The listing builds one solid part. Answer for the finished solid, in the listing's coordinates (mm). Give positions to 0.01 mm unless a question says otherwise; leave off trailing zeros. Write each loop counter-clockwise with the first axis right and the second up, starting at its lowest first coordinate (ties: lowest second). Pieces come first, ordered by that corner, then holes. Notation, with made-up numbers: M 50,47 L 58,47 A15 cw 58,75 Z; hole C 4.5,66 d8. An arc over 180 degrees is marked long. Answer as a JSON object with one key per item and string values.
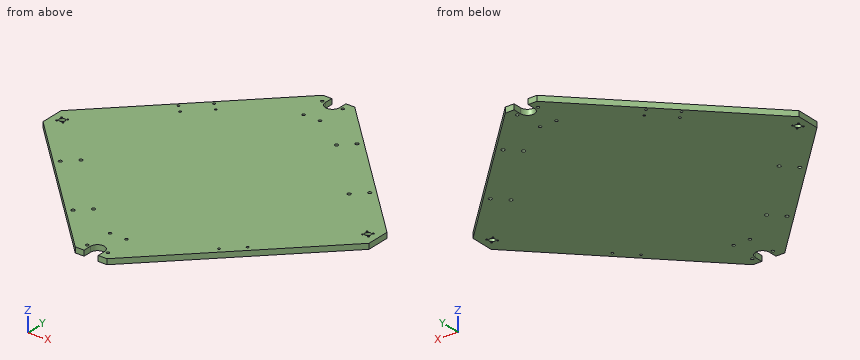
Autodesk Inventor part; units mm, degrees
ref_plane "Work Plane1" through (0, 0, 0) normal (0, 0, 1) x (1, 0, 0)
ref_plane "YZ Plane" through (0, 0, 0) normal (1, 0, 0) x (0, 1, 0)
ref_plane "XZ Plane" through (0, 0, 0) normal (0, 1, 0) x (-1, 0, 0)
sketch "Sketch2" plane through (0, 0, 0) normal (0, 0, 1) x (1, 0, 0)
  circle A0 centre (0, 277.5) radius 8 construction
  circle A1 centre (0, 277.5) radius 13
  circle A2 centre (0, 277.5) radius 10.5 construction
  line L0 (25, 287.5) -> (-25, 287.5) construction
  line L1 (-25, 287.5) -> (-25, 222.5) construction
  line L2 (-25, 222.5) -> (25, 222.5) construction
  line L3 (25, 222.5) -> (25, 287.5) construction
  circle A3 centre (15, 228.5) radius 2.7
  circle A4 centre (-15, 228.5) radius 2.7
  circle A5 centre (-19, 277.5) radius 2.7
  circle A6 centre (19, 277.5) radius 2.7
  circle A7 centre (0, -277.5) radius 8 construction
  circle A8 centre (0, -277.5) radius 13
  circle A9 centre (0, -277.5) radius 10.5 construction
  line L4 (25, -287.5) -> (-25, -287.5) construction
  line L5 (-25, -287.5) -> (-25, -222.5) construction
  line L6 (-25, -222.5) -> (25, -222.5) construction
  line L7 (25, -222.5) -> (25, -287.5) construction
  circle A10 centre (-15, -228.5) radius 2.7
  circle A11 centre (15, -228.5) radius 2.7
  circle A12 centre (-19, -277.5) radius 2.7
  circle A13 centre (19, -277.5) radius 2.7
  line L8 (10.5, -277.5) -> (10.5, -287.5) construction
  line L9 (-10.5, -277.5) -> (-10.5, -287.5) construction
  line L10 (10.5, 277.5) -> (10.5, 287.5) construction
  line L11 (-10.5, 277.5) -> (-10.5, 287.5) construction
  circle A14 centre (281.7, 0) radius 5.25
  circle A15 centre (-281.7, 0) radius 5.25
  line L12 (0, -321.7336) -> (321.7336, 0)
  line L13 (321.7336, 0) -> (0, 321.7336)
  line L14 (0, 321.7336) -> (-321.7336, 0)
  line L15 (-321.7336, 0) -> (0, -321.7336)
  line L16 (0, -321.7336) -> (0, 321.7336) construction
  line L17 (321.7336, 0) -> (-321.7336, 0) construction
  line L18 (0, -321.7336) -> (455, -321.7336) construction
  line L19 (300.5, 21.2336) -> (300.5, -21.2336)
  line L20 (-300.5, 21.2336) -> (-300.5, -21.2336)
  line L21 (-24.2336, 297.5) -> (24.2336, 297.5) construction
  line L22 (-29.2336, 292.5) -> (29.2336, 292.5)
  line L23 (-24.2336, -297.5) -> (24.2336, -297.5) construction
  line L24 (-29.2336, -292.5) -> (29.2336, -292.5)
  line L25 (-9.5, 297.5) -> (-3.976, 284.442) construction
  line L26 (9.5, 297.5) -> (3.976, 284.442) construction
  line L27 (-14.929, 297.5) -> (-9.9883, 285.8207)
  line L28 (14.929, 297.5) -> (9.9883, 285.8207)
  line L29 (-9.5, -297.5) -> (-3.976, -284.442) construction
  line L30 (9.5, -297.5) -> (3.976, -284.442) construction
  line L31 (14.929, -297.5) -> (9.9883, -285.8207)
  line L32 (-14.929, -297.5) -> (-9.9883, -285.8207)
  line L33 (13, 277.5) -> (13, 292.5)
  line L34 (-13, 277.5) -> (-13, 292.5)
  line L35 (-13, -277.5) -> (-13, -292.5)
  line L36 (13, -277.5) -> (13, -292.5)
  line L37 (281.7, 0) -> (287.3569, 5.6569) construction
  line L38 (281.7, 0) -> (289.7, 0) construction
  circle A16 centre (287.3569, 5.6569) radius 1.6
  circle A17 centre (276.0431, 5.6569) radius 1.6
  circle A18 centre (276.0431, -5.6569) radius 1.6
  circle A19 centre (287.3569, -5.6569) radius 1.6
  line L39 (-281.7, 0) -> (-287.3569, 5.6569) construction
  circle A20 centre (-287.3569, 5.6569) radius 1.6
  circle A21 centre (-287.3569, -5.6569) radius 1.6
  circle A22 centre (-276.0431, -5.6569) radius 1.6
  circle A23 centre (-276.0431, 5.6569) radius 1.6
  point P0 (0, 0)
  point P1 (-12.8138, -292.5)
  point P2 (12.8138, -292.5)
  point P3 (12.8138, 292.5)
  point P4 (-12.8138, 292.5)
  point P5 (300.5, 292.5)
  point P6 (300.5, -292.5)
  point P7 (-300.5, -292.5)
  point P8 (-300.5, 292.5)
  dimension "d349" = 450
  dimension "d350" = 45
  dimension "d353" = 40
  dimension "d354" = 10
  dimension "d355" = 10
  dimension "d358" = 40
  dimension "d359" = 10
  dimension "d360" = 10
  dimension "d361" = 6.2
  dimension "d362" = 75
  dimension "d363" = 5
  dimension "d364" = 6.2
  dimension "d365" = 5
  dimension "d366" = 75
  dimension "d367" = 450
  dimension "d368" = 45
  dimension "d369" = 6.2
  dimension "d370" = 5
  dimension "d371" = 75
  dimension "d372" = 6.2
  dimension "d373" = 5
  dimension "d374" = 75
  dimension "d256" = 16
  dimension "d257" = 0
  dimension "d258" = 277.5
  dimension "d259" = 26
  dimension "d260" = 21
  dimension "d261" = 50
  dimension "d262" = 10
  dimension "d263" = 65
  dimension "d265" = 50
  dimension "d266" = 25
  dimension "d267" = 5.4
  dimension "d268" = 5.4
  dimension "d269" = 5.4
  dimension "d270" = 5.4
  dimension "d271" = 6
  dimension "d272" = 10
  dimension "d273" = 6
  dimension "d274" = 10
  dimension "d275" = 6
  dimension "d276" = 10
  dimension "d277" = 6
  dimension "d278" = 10
  dimension "d279" = 0
  dimension "d280" = 277.5
  dimension "d281" = 26
  dimension "d282" = 16
  dimension "d283" = 21
  dimension "d284" = 50
  dimension "d285" = 10
  dimension "d286" = 65
  dimension "d287" = 25
  dimension "d288" = 5.4
  dimension "d289" = 5.4
  dimension "d290" = 5.4
  dimension "d291" = 5.4
  dimension "d292" = 6
  dimension "d293" = 10
  dimension "d294" = 6
  dimension "d295" = 10
  dimension "d296" = 10
  dimension "d297" = 6
  dimension "d298" = 10
  dimension "d299" = 6
  dimension "d300" = 10.5
  dimension "d301" = 0
  dimension "d302" = 281.7
  dimension "d310" = 10.5
  dimension "d311" = 0
  dimension "d312" = 281.7
  dimension "d320" = 455
  dimension "d321" = 45
  dimension "d322" = 455
  dimension "d323" = 18.8
  dimension "d324" = 18.8
  dimension "d325" = 20
  dimension "d326" = 15
  dimension "d327" = 20
  dimension "d328" = 15
  dimension "d329" = 67.07
  dimension "d330" = 67.07
  dimension "d331" = 9.5
  dimension "d332" = 9.5
  dimension "d333" = 67.07
  dimension "d334" = 67.07
ref_plane "Work Plane1" through (0, 0, 0) normal (0, 0, 1) x (1, 0, 0)
sketch "Sketch3" plane through (0, 0, 0) normal (0, 0, 1) x (1, 0, 0)
  line L0 (-159.099, -159.099) -> (159.099, 159.099)
  line L1 (-159.099, -159.099) -> (290.901, -159.099) construction
  line L2 (279.2843, 34.9264) -> (34.9264, 279.2843)
  line L3 (34.9264, 279.2843) -> (6.6421, 251)
  line L4 (6.6421, 251) -> (251, 6.6421)
  line L5 (251, 6.6421) -> (279.2843, 34.9264)
  line L6 (279.2843, 34.9264) -> (6.6421, 251) construction
  line L7 (34.9264, 279.2843) -> (251, 6.6421) construction
  circle A0 centre (19, 277.5) radius 2.7
  circle A1 centre (15, 228.5) radius 2.7
  line L8 (-34.9264, -279.2843) -> (-279.2843, -34.9264)
  line L9 (-279.2843, -34.9264) -> (-251, -6.6421)
  line L10 (-251, -6.6421) -> (-6.6421, -251)
  line L11 (-6.6421, -251) -> (-34.9264, -279.2843)
  line L12 (-34.9264, -279.2843) -> (-251, -6.6421) construction
  line L13 (-279.2843, -34.9264) -> (-6.6421, -251) construction
  circle A2 centre (-15, -228.5) radius 2.7
  circle A3 centre (-19, -277.5) radius 2.7
  circle A4 centre (-79.3236, -185.3896) radius 3.1
  circle A5 centre (-100.5368, -206.6028) radius 3.1
  circle A6 centre (-185.3896, -79.3236) radius 3.1
  circle A7 centre (-206.6028, -100.5368) radius 3.1
  line L14 (-159.099, 159.099) -> (159.099, -159.099)
  line L15 (300.5, -21.2336) -> (29.2336, -292.5)
  line L16 (-159.099, 159.099) -> (290.901, 159.099) construction
  circle A8 centre (206.6028, 100.5368) radius 3.1
  circle A9 centre (185.3896, 79.3236) radius 3.1
  circle A10 centre (100.5368, 206.6028) radius 3.1
  circle A11 centre (79.3236, 185.3896) radius 3.1
  point P0 (0, 0)
  point P1 (142.9632, 142.9632)
  point P2 (-142.9632, -142.9632)
  point P3 (29.2336, -292.5)
  dimension "d349" = 450
  dimension "d350" = 45
  dimension "d353" = 40
  dimension "d354" = 10
  dimension "d355" = 10
  dimension "d358" = 40
  dimension "d359" = 10
  dimension "d360" = 10
  dimension "d361" = 6.2
  dimension "d362" = 75
  dimension "d363" = 5
  dimension "d364" = 6.2
  dimension "d365" = 5
  dimension "d366" = 75
  dimension "d367" = 450
  dimension "d368" = 45
  dimension "d369" = 6.2
  dimension "d370" = 5
  dimension "d371" = 75
  dimension "d372" = 6.2
  dimension "d373" = 5
  dimension "d374" = 75
extrude "Extrusion12" add sketch "Sketch2" against normal blind 10 contours L33 L22 L13 L19 L12 L24 L36 A8 L35 L15 L20 L14 L34 A1
hole "Hole2" at (100.5368, 206.6028, 0) at (79.3236, 185.3896, 0) at (206.6028, 100.5368, 0) at (185.3896, 79.3236, 0) at (-79.3236, -185.3896, 0) at (-100.5368, -206.6028, 0) at (-185.3896, -79.3236, 0) at (-206.6028, -100.5368, 0) direction (0, 0, -1) diameter 6.2 end through all
sketch "Sketch4" plane through (0, 0, 0) normal (0, 0, 1) x (1, 0, 0)
  line L0 (-160.8668, -160.8668) -> (160.8668, 160.8668)
  line L1 (29.2336, 292.5) -> (300.5, 21.2336)
  line L2 (-160.8668, -160.8668) -> (294.1332, -160.8668) construction
  line L3 (160.8668, -160.8668) -> (-160.8668, 160.8668)
  line L4 (-175.0089, 138.2394) -> (-138.2394, 175.0089) construction
  line L5 (-138.2394, 175.0089) -> (-125.5115, 162.281) construction
  line L6 (-125.5115, 162.281) -> (-162.281, 125.5115) construction
  line L7 (-162.281, 125.5115) -> (-175.0089, 138.2394) construction
  line L8 (-175.0089, 138.2394) -> (-125.5115, 162.281) construction
  line L9 (-138.2394, 175.0089) -> (-162.281, 125.5115) construction
  circle A0 centre (-138.2394, 175.0089) radius 2.1
  circle A1 centre (-125.5115, 162.281) radius 2.1
  circle A2 centre (-175.0089, 138.2394) radius 2.1
  circle A3 centre (-162.281, 125.5115) radius 2.1
  circle A4 centre (138.9465, -168.645) radius 2.1
  circle A5 centre (168.645, -138.9465) radius 2.1
  line L10 (138.9465, -168.645) -> (168.645, -138.9465) construction
  point P0 (0, 0)
  point P1 (-150.2602, 150.2602)
  point P2 (153.7957, -153.7957)
  dimension "d406" = 455
  dimension "d407" = 45
  dimension "d413" = 52
  dimension "d415" = 18
  dimension "d416" = 221.5
  dimension "d417" = 4.2
  dimension "d418" = 4.2
  dimension "d419" = 4.2
  dimension "d420" = 4.2
  dimension "d421" = 4.2
  dimension "d422" = 4.2
  dimension "d423" = 42
  dimension "d424" = 217.5
hole "Hole3" at (-175.0089, 138.2394, 0) at (-162.281, 125.5115, 0) at (-125.5115, 162.281, 0) at (-138.2394, 175.0089, 0) at (138.9465, -168.645, 0) at (168.645, -138.9465, 0) direction (0, 0, -1) diameter 4.2 end through all
equation "\"dist_rails\" = 555"
equation "\"dist_leadscrews\" = 563.4"
equation "\"diam_leadscrew_hole\" = 10.5"
equation "\"z_plate_width\" = 455"
equation "\"delta\" = 5"
equation "\"rail_angle\" = 67.07deg"
equation "\"rail_D\" = 9.5"
equation "\"rail_diam\" = 16"
properties part number "z_plate" material "Aluminum 6061"
1. A cutting plane is placed at B-B, the plane x = 261. Give the vertices of the cut face in (y, z).
Verdict:
{"outline": "M -60.73,-10 L 60.73,-10 L 60.73,0 L -60.73,0 Z"}
2. A cutting plane is placed at A-A, the plane z = -7.5. Count the separate pieces of the cut face and the enclosed holes in it, plus the area to 3 significant figures.
Verdict:
{"separate pieces": "1", "enclosed holes": "32", "area": "202,000 mm2"}
3. A cutting plane is placed at C-C, the plane x = 154. Give the vertices of the cut face in (y, z).
Verdict:
{"outline": "M -167.73,-10 L 167.73,-10 L 167.73,0 L -167.73,0 Z"}
4. Flat-ended cylindrical pins translate along their axes: pin 1 (2 mm diameter, centred on y = -148, z = -7.5, fed in from +X); pin 2 (3 mm diameter, centred on y = -83, z = -4.5, fed in from -X). Find the tip coordinate at first contact, or state that the pin passes through.
Verdict:
{"pin 1": "stops at x = 174.73", "pin 2": "stops at x = -240.23"}
5. Consider line 1 along Y through (x, z) = (15, -2); line 2 along X through (y, z) = (-277.5, -5.75); line 3 along X through (y, z) = (228.5, -2). Determine where each line is inside the solid, lowest interval first.
Verdict:
{"line 1": "y = -292.5 to -231.2, -225.8 to 225.8, 231.2 to 292.5", "line 2": "x = -44.23 to -21.7, -16.3 to -13, 13 to 16.3, 21.7 to 44.23", "line 3": "x = -93.23 to -17.7, -12.3 to 12.3, 17.7 to 93.23"}
